```python
from build123d import *

# Parameters (mm, degrees)
SKETCH_1_W               = 24
SKETCH_1_H               = 38
EXTRUDE_1_DEPTH          = 5
SKETCH_2_R               = 2.75
CUT_EXTRUDE_1_DEPTH      = 10.25
CUT_EXTRUDE_2_DEPTH      = 24.021728866
CUT_EXTRUDE_2_DEPTH_BACK = 24.021728866
SKETCH_3_R               = 1
CUT_EXTRUDE_3_DEPTH      = 0.5
SKETCH_5_R               = 1.75
CUT_EXTRUDE_4_DEPTH      = 24.021728866
FILLET_1_R               = 3
FILLET_2_R               = 3
SKETCH_6_R               = 1.5
CUT_EXTRUDE_5_DEPTH      = 8
FILLET_3_R               = 0.5
SKETCH_7_R               = 1.25
CUT_EXTRUDE_6_DEPTH      = 24.02172894
CUT_EXTRUDE_9_DEPTH      = 3
CUT_EXTRUDE_10_DEPTH     = 2
FILLET_4_R               = 0.5


with BuildPart() as part:
    # Эскиз1 → Бобышка-Вытянуть1 (new body)
    with BuildSketch(Plane(origin=(0, 0, 0), x_dir=(1, 0, 0), z_dir=(0, 1, 0))):
        Rectangle(SKETCH_1_W, SKETCH_1_H)
    extrude(amount=EXTRUDE_1_DEPTH)

    # Эскиз2 → Вырез-Вытянуть1 (cut, symmetric)
    with BuildSketch(Plane(origin=(0, 0, 0), x_dir=(0, 0, -1), z_dir=(1, 0, 0))):
        with Locations((-12.75, 5)):
            Circle(SKETCH_2_R)
        with Locations((12.75, 5)):
            Circle(SKETCH_2_R)
    extrude(amount=CUT_EXTRUDE_1_DEPTH, both=True, mode=Mode.SUBTRACT)

    # Эскиз3 → Вырез-Вытянуть2 (cut, two sides: drawn at the far end of the back side and taken through both)
    with BuildSketch(Plane(origin=(0, 0, 0), x_dir=(0, 0, -1), z_dir=(1, 0, 0)).offset(-CUT_EXTRUDE_2_DEPTH_BACK)):
        with Locations((-12.75, 5)):
            Circle(SKETCH_3_R)
        with Locations((12.75, 5)):
            Circle(SKETCH_3_R)
    extrude(amount=CUT_EXTRUDE_2_DEPTH + CUT_EXTRUDE_2_DEPTH_BACK, mode=Mode.SUBTRACT)

    # Эскиз4 → Вырез-Вытянуть3 (cut)
    with BuildSketch(Plane(origin=(0, 5, 0), x_dir=(1, 0, 0), z_dir=(0, 1, 0))):
        with BuildLine():
            Line((4, 7), (-12, 7))
            Line((-12, 7), (-12, 5.5))
            Line((-12, 5.5), (-0.330127019, 5.5))
            ThreePointArc((-0.330127019, 5.5), (-3, 0), (-0.330127019, -5.5))
            Line((-0.330127019, -5.5), (-12, -5.5))
            Line((-12, -5.5), (-12, -7))
            Line((-12, -7), (4, -7))
            ThreePointArc((4, -7), (8.677071733, -5.208166664), (10.959705454, -0.75))
            Line((10.959705454, -0.75), (12, -0.75))
            Line((12, -0.75), (12, 0.75))
            Line((12, 0.75), (10.959705454, 0.75))
            ThreePointArc((10.959705454, 0.75), (8.677071733, 5.208166664), (4, 7))
        make_face()
    extrude(amount=-CUT_EXTRUDE_3_DEPTH, mode=Mode.SUBTRACT)

    # Эскиз5 → Вырез-Вытянуть4 (cut, through all)
    with BuildSketch(Plane(origin=(0, 5, 0), x_dir=(1, 0, 0), z_dir=(0, 1, 0))):
        with Locations(Location((4, 0, 0), (0, 0, 270))):
            Circle(SKETCH_5_R)
        with Locations(Location((-7, 0, 0), (0, 0, 270))):
            Circle(SKETCH_5_R)
    extrude(amount=-CUT_EXTRUDE_4_DEPTH, mode=Mode.SUBTRACT)

    # Скругление1
    fillet_1_edges = [part.edges().sort_by_distance(p)[0] for p in [
        (-0.330127019, 4.75, 5.5),
        (-0.330127019, 4.75, -5.5),
    ]]
    fillet(fillet_1_edges, radius=FILLET_1_R)

    # Скругление2
    fillet_2_edges = [part.edges().sort_by_distance(p)[0] for p in [
        (12, 2.5, 19),
        (-12, 2.5, 19),
        (-12, 2.5, -19),
        (12, 2.5, -19),
    ]]
    fillet(fillet_2_edges, radius=FILLET_2_R)

    # Эскиз6 → Вырез-Вытянуть5 (cut)
    with BuildSketch(Plane.ZY.offset(12)):
        with Locations((0, 5)):
            Circle(SKETCH_6_R)
    extrude(amount=-CUT_EXTRUDE_5_DEPTH, mode=Mode.SUBTRACT)

    # Скругление3
    fillet_3_edges = [part.edges().sort_by_distance(p)[0] for p in [
        (10.959705454, 4.75, -0.75),
        (10.959705454, 4.75, 0.75),
    ]]
    fillet(fillet_3_edges, radius=FILLET_3_R)

    # Эскиз7 → Вырез-Вытянуть6 (cut, through all)
    with BuildSketch(Plane(origin=(0, 5, 0), x_dir=(1, 0, 0), z_dir=(0, 1, 0))):
        with Locations(Location((-7, 17, 0), (0, 0, 270))):
            Circle(SKETCH_7_R)
        with Locations(Location((7, 17, 0), (0, 0, 270))):
            Circle(SKETCH_7_R)
        with Locations(Location((7, -17, 0), (0, 0, 270))):
            Circle(SKETCH_7_R)
        with Locations(Location((-7, -17, 0), (0, 0, 270))):
            Circle(SKETCH_7_R)
    extrude(amount=-CUT_EXTRUDE_6_DEPTH, mode=Mode.SUBTRACT)

    # Эскиз9 → Вырез-Вытянуть9 (cut)
    with BuildSketch(Plane.XZ):
        Polygon((-7, 3.290896534), (-9.85, 1.645448267), (-9.85, -1.645448267), (-7, -3.290896534), (-4.15, -1.645448267), (-4.15, 1.645448267), align=None)
        Polygon((6.85, -1.645448267), (6.85, 1.645448267), (4, 3.290896534), (1.15, 1.645448267), (1.15, -1.645448267), (4, -3.290896534), align=None)
    extrude(amount=-CUT_EXTRUDE_9_DEPTH, mode=Mode.SUBTRACT)

    # Эскиз10 → Вырез-Вытянуть10 (cut)
    with BuildSketch(Plane.XZ):
        Polygon((8.198001809, 14.925), (5.801998191, 14.925), (4.603996383, 17), (5.801998191, 19.075), (8.198001809, 19.075), (9.396003617, 17), align=None)
        Polygon((-5.801998191, 14.925), (-4.603996383, 17), (-5.801998191, 19.075), (-8.198001809, 19.075), (-9.396003617, 17), (-8.198001809, 14.925), align=None)
        Polygon((9.396003617, -17), (8.198001809, -14.925), (5.801998191, -14.925), (4.603996383, -17), (5.801998191, -19.075), (8.198001809, -19.075), align=None)
        Polygon((-8.198001809, -14.925), (-5.801998191, -14.925), (-4.603996383, -17), (-5.801998191, -19.075), (-8.198001809, -19.075), (-9.396003617, -17), align=None)
    extrude(amount=-CUT_EXTRUDE_10_DEPTH, mode=Mode.SUBTRACT)

    # Скругление4
    # the kernel refuses this fillet: 0.5 mm, written as the material it takes off along each edge
    with BuildSketch(Plane(origin=(-8.241303079, 2, 19), x_dir=(-0.9999949104209014, 0, -0.003190475245701581), z_dir=(0, -1, 0)), Plane(origin=(8.241303079, 2, -19), x_dir=(0.9999949104209014, 0, 0.003190475245705545), z_dir=(0, -1, 0))) as fillet_4_piece_1:
        with BuildLine():
            CenterArc((0.868988605, 0.499594021), FILLET_4_R, 149.817198924, 122.491852834)
            Line((0.436775726, 0.750974265), (0.393554438, 0.77611229))
            Line((0.393554438, 0.77611229), (-0.043221288, 0.025138024))
            Line((-0.043221288, 0.025138024), (-0.000159524, -0.049999746))
            ThreePointArc((-0.000159524, -0.049999746), (0.758533536, -0.052420349), (0.891147911, -0.049959402))
            Line((0.891147911, -0.049959402), (0.889133429, 0))
        make_face()
    extrude(amount=4.222833572, mode=Mode.SUBTRACT)
    with BuildSketch(Plane(origin=(-5.758696921, -2.165063509, 19), x_dir=(1, 0, 0), z_dir=(0, 1, 0)), Plane(origin=(5.758696921, -2.165063509, -19), x_dir=(-1, 0, 0), z_dir=(0, 1, 0))) as fillet_4_piece_2:
        with BuildLine():
            CenterArc((FILLET_4_R * 1.73205080757, FILLET_4_R), FILLET_4_R, 150, 120)
            Line((FILLET_4_R * 0.866025403784, FILLET_4_R * 1.5), (0, 0))
            Line((0, 0), (FILLET_4_R * 1.73205080757, 0))
        make_face()
    extrude(amount=4.165063509, mode=Mode.SUBTRACT)
    with BuildSketch(Plane(origin=(-5.758696921, -2.165063509, -19), x_dir=(1, 0, 0), z_dir=(0, 1, 0)), Plane(origin=(5.758696921, -2.165063509, 19), x_dir=(-1, 0, 0), z_dir=(0, 1, 0))) as fillet_4_piece_3:
        with BuildLine():
            CenterArc((FILLET_4_R * 1.73205080757, -FILLET_4_R), FILLET_4_R, 90, 120)
            Line((FILLET_4_R * 0.866025403784, -FILLET_4_R * 1.5), (0, 0))
            Line((0, 0), (FILLET_4_R * 1.73205080757, 0))
        make_face()
    extrude(amount=4.165063509, mode=Mode.SUBTRACT)
    with BuildSketch(Plane(origin=(-8.241303079, 2, -19), x_dir=(-0.9999949104209014, 0, 0.0031904752457015684), z_dir=(0, -1, 0)), Plane(origin=(8.241303079, 2, 19), x_dir=(0.9999949104209014, 0, -0.003190475245701575), z_dir=(0, -1, 0))) as fillet_4_piece_4:
        with BuildLine():
            CenterArc((0.868988605, -0.499594021), FILLET_4_R, 87.690948243, 122.491852834)
            Line((0.436775726, -0.750974265), (0.393554438, -0.77611229))
            Line((0.393554438, -0.77611229), (-0.043221288, -0.025138024))
            Line((-0.043221288, -0.025138024), (-0.000159524, 0.049999746))
            ThreePointArc((-0.000159524, 0.049999746), (0.758533536, 0.052420349), (0.891147911, 0.049959402))
            Line((0.891147911, 0.049959402), (0.889133429, 0))
        make_face()
    extrude(amount=4.222833572, mode=Mode.SUBTRACT)


solid = part.part
```
Read the model definition and answer for the solid it produces. Units are mm, in the model's axes. A direction names the side the tool comes from. Coordinates: 2 decimals unless noted, no trailing zeros. Write each loop counter-clockwise with the first axis right and the second up, starting at its lowest first coordinate (ties: lowest second). Pieces come first, ordered by that corner, then holes. Notation, with made-up numbers: (-37.5, -16) -> (-20.5, -16) arc R8 ccw to (-20.5, -1) -> close; hole circle Ø5 at (22.25, -35.75). An arc over 180 degrees is marked (long way). Return JSON: item names as keys, results as strings.
1. Find the intervals of material crossed by line 1 along X through (y, z) = (2.1, 1); line 2 along X through (y, z) = (3.4, 0); line 3 along Z through (x, y) = (-5, 1.4), in increasing order. Write a range as from..to.
Found:
{"line 1": "-12..-9.85, -4.15..1.15, 6.85..12", "line 2": "-12..-8.75, -5.25..2.25, 5.75..12", "line 3": "-18.99..-17.69, -16.31..-2.14, 2.14..16.31, 17.69..18.99"}
2. A cutting plane is placed at B-B (z = -12.75). Determine the outline of the cut face in (x, y), and give its area (3 significant figures).
Found:
{"outline": "(-12, 0) -> (12, 0) -> (12, 4) -> (10.25, 4) -> (10.25, 2.25) -> (-10.25, 2.25) -> (-10.25, 4) -> (-12, 4) -> close", "area": "60.1 mm2"}
3. A cutting plane is placed at D-D (z = 14.5). Determine the outline of the cut face in (x, y).
Found:
{"outline": "(-12, 0) -> (12, 0) -> (12, 5) -> (10.25, 5) -> (10.25, 2.88) -> (-10.25, 2.88) -> (-10.25, 5) -> (-12, 5) -> close"}
4. Determine the mould class of faces 1 (the face through (-12, 2, 0)), 2 (the face through (-9.85, 1, 0)), 3 (the face through (2.595, 1.479, 2.48)), 4 (the face through (0, 5, -17)) for opening direction X: pulls with the +X half, pulls with the -X half, needs draft (parallel to the pull), parting line crosses it, or undercut.
Found:
{"face 1": "pulls with the -X half", "face 2": "undercut", "face 3": "undercut", "face 4": "needs draft"}
5. A cutting plane is placed at C-C (y = 0.7). Give the number of separate pieces and of enclosed holes in the cut face, and give its area (3 significant figures).
Found:
{"separate pieces": "1", "enclosed holes": "2", "area": "788 mm2"}
6. A cutting plane is placed at A-A (z = 0). Determine the outline of the cut face in (x, y), and give its area (3 significant figures).
Found:
{"outline": "(-12, 0) -> (-9.85, 0) -> (-9.85, 3) -> (-8.75, 3) -> (-8.75, 3.5) -> (-12, 3.5) -> close; (-5.25, 3) -> (-4.15, 3) -> (-4.15, 0) -> (1.15, 0) -> (1.15, 3) -> (2.25, 3) -> (2.25, 4.5) -> (-3, 4.5) -> (-3, 5) -> (-4, 5) -> (-4, 3.5) -> (-5.25, 3.5) -> close; (5.75, 3) -> (6.85, 3) -> (6.85, 0) -> (12, 0) -> (12, 4.5) -> (5.75, 4.5) -> close", "area": "59.3 mm2"}
7. Each of these flat-tipped pins is pushed along its axis until it touches: P1, Ø0.6, axis at x = 7, y = 1.5, coming from the -Z side (3 decimals); P2, Ø2, axis at x = 7, z = 16.5, coming from the -Y side; P3, Ø1, axis at x = -7.5, z = 1, coming from the -Y side; P4, Ø1, axis at x = 7, z = 1, coming from the +Y side. Where does it stop, or does it pass through?
Found:
{"P1": "z = -14.925", "P2": "y = 2", "P3": "through", "P4": "y = 4.5"}
8. A tool of negligible diameter and unlimited length cuts with its end or side. For faces 5 (the face through (5.21, 0.99, 15.95)), 6 (the face through (11.14, 2.54, 18.1)), from which of +Z, -Z, +X, -X, +Y, -Y can it reach the whole face along a straight path? Write none if from no direction.
Found:
{"face 5": "-Y", "face 6": "+Z, +X, +Y, -Y"}
